Input: dimensioned drawing with shaded views. Units: mm. Origin: part minimum x, y, z. A direction names the side the tool comes from. Give positions to 0.01 mm unless a question says otherwise; leave off trailing zeros. Write each loop counter-clockwise with the first axis right and the second up, starting at its lowest first coordinate (ties: lowest second). Pieces come first, ordered by that corner, then holes. Notation, with made-up numbers: M 27.25,57.5 L 71.25,57.5 A34 ccw 71.25,91.5 Z; hole C 25.25,25 d3. An arc over 180 degrees is marked long. Use CSV: the item, a comma, the result in double quotes. Start each with the question number.
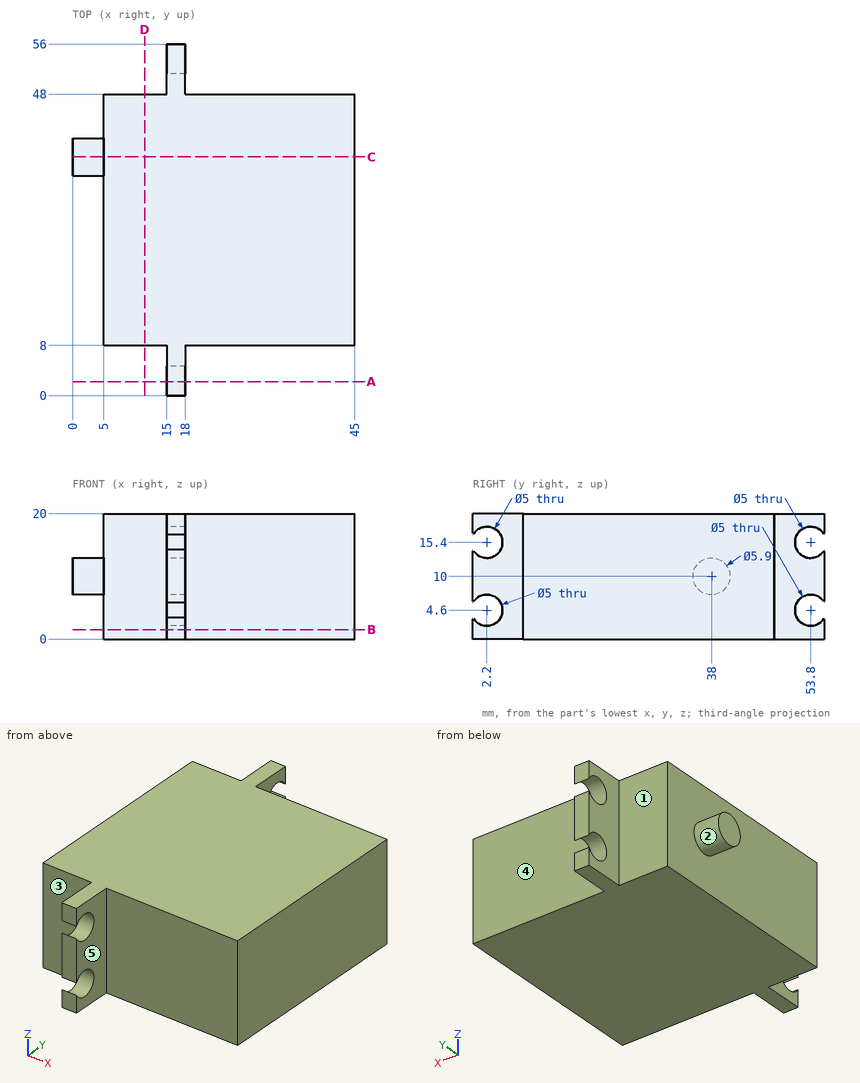
Item 1: Section B-B (z = 1.5). Return the cut outline in (x, y), plus the area to 3 significant figures.
Item 2: Material intervals for probe 1 along Z at (x, y) = (16.85, 53.8); probe 2 along Z at (x, y) = (16, 53); probe 3 along X at (y, z) = (19, 14.25), sorted ascending.
Item 3: Set-up query: the marked faces 1, 2, 3, 4 and 5. Return all of +Z, -Z, +X, -X, +Y, -Y with unobstructed straight access to the full face (end or side cutting, diameter ignored); none if empty.
Item 4: Section C-C (y = 38). Return the cut outline in (x, z).
Item 5: Contact query for flat-ended pins moving along their axis: pin 1 Ø6 at (x, z) = (35.5, 5.5) entering from +Y; pin 2 Ø1.5 at (y, z) = (19, 10.5) entering from -X; pin 3 Ø10 at (x, z) = (28.5, 12) entering from -Y. Output: stop coordinate, or through.
Item 6: Section A-A (y = 2.2). Return the cut outline in (x, z), plus the area to 3 significant figures.
Item 7: Section D-D (x = 11.5). Return the cut outline in (y, z), plus the area to 3 significant figures.
Output values:
1,outline,"M 5,8 L 15,8 L 15,0 L 18,0 L 18,8 L 45,8 L 45,48 L 18,48 L 18,56 L 15,56 L 15,48 L 5,48 Z"
1,area,"1,650 mm2"
2,probe 1,"z = 0 to 2.1, 7.1 to 12.9, 17.9 to 20"
2,probe 2,"z = 0 to 2.23, 6.97 to 13.03, 17.77 to 20"
2,probe 3,"x = 5 to 45"
3,face 1,"+Z, -Z, -X, +Y"
3,face 2,"-X"
3,face 3,"+Z, -Z, -X, -Y"
3,face 4,"+Z, -Z, +X, +Y"
3,face 5,"+Z, -Z, +X, -Y"
4,outline,"M 0,7.05 L 5,7.05 L 5,0 L 45,0 L 45,20 L 5,20 L 5,12.95 L 0,12.95 Z"
5,pin 1,"stops at y = 48"
5,pin 2,"stops at x = 5"
5,pin 3,"stops at y = 8"
6,outline,"M 15,0 L 18,0 L 18,2.1 L 15,2.1 Z; M 15,7.1 L 18,7.1 L 18,12.9 L 15,12.9 Z; M 15,17.9 L 18,17.9 L 18,20 L 15,20 Z"
6,area,"30.0 mm2"
7,outline,"M 8,0 L 48,0 L 48,20 L 8,20 Z"
7,area,"800 mm2"
